Autodesk Inventor part; units mm, degrees
ref_plane "YZ Plane" through (0, 0, 0) normal (1, 0, 0) x (0, 1, 0)
ref_plane "XZ Plane" through (0, 0, 0) normal (0, 1, 0) x (-1, 0, 0)
ref_plane "XY Plane" through (0, 0, 0) normal (0, 0, 1) x (1, 0, 0)
sketch "Sketch1" plane through (0, 0, 0) normal (0, 1, 0) x (-1, 0, 0)
  circle A0 centre (0, 0) radius 5
  circle A1 centre (0, 0) radius 1.5
  dimension "d0" = 10
  dimension "d1" = 3
extrude "Extrusion1" add sketch "Sketch1" along normal blind 5.5
chamfer "Chamfer1" distance 2 angle 45 1 edges at (1.5, 5.5, 0)
fillet "Fillet1" radius 2 1 edges at (1.5, 3.5, 0)
fillet "Fillet2" radius 1.6 1 edges at (3.5, 5.5, 0)
fillet "Fillet3" radius 1 1 edges at (5, 5.5, 0)
fillet "Fillet4" radius 0.3 1 edges at (5, 0, 0)
fillet "Fillet5" radius 0.3 1 edges at (1.5, 0, 0)
properties part number "TransformerLug"
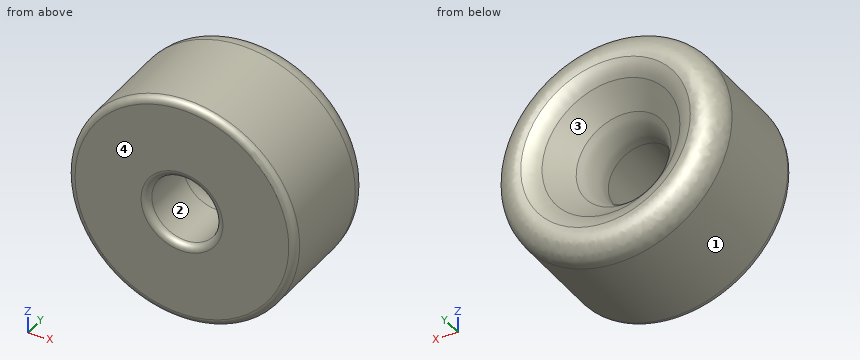
Design review of the part built by this model. Coordinates are the model's own, in mm. Face numbers are marked on the shaded views. Coordinates: 2 decimals unless noted, no trailing zeros. Order: outer loops, then holes, each group sorted by start corner. A loop starts at its lowest first (then second) coordinate and runs counter-clockwise, first axis right, second up. Notation, with made-up numbers: M 18.5,16 L 51.5,16 A25 ccw 51.5,48 Z; hole C 15.5,36 d9. An arc over 180 degrees is marked long. Use a Markdown table: item, result.
(1) Add section A-A (y = 1.7). Give the boundary of the cut face in (x, z).
Worked answers:
| item | result |
|---|---|
| outline | C 0,0 d10; hole C 0,0 d3 |
(2) Wall thickness on probe 1 along Z at (x, y) = (0, 1.5); probe 2 along Y at (x, z) = (3, -2.75): over which ranges is each line inside the solid? List them lowest first.
Worked answers:
| item | result |
|---|---|
| probe 1 | z = -5 to -1.5, 1.5 to 5 |
| probe 2 | y = 0 to 5.48 |
(3) For P1, Ø1.5, axis at x = -2.5, y = 4, coming from the -Z side; P2, Ø1.5, axis at x = -3.5, y = 5, coming from the +Z side; P3, Ø1.5, axis at x = -1, z = 1, coming from the +Y side, all flat-tipped, find the tip position at first contact; note any pin that passes through.
Worked answers:
| item | result |
|---|---|
| P1 | stops at z = -4.68 |
| P2 | stops at z = 4.1 |
| P3 | stops at y = 4.16 |
(4) Draft analysis for pull direction Z (two halves, no side actions). For the marked faces 1, 2, 3 and 4, state which applies: released by +Z, released by -Z, zero draft, split by the parting line, or undercut.
Worked answers:
| item | result |
|---|---|
| face 1 | split by the parting line |
| face 2 | undercut |
| face 3 | undercut |
| face 4 | zero draft |
